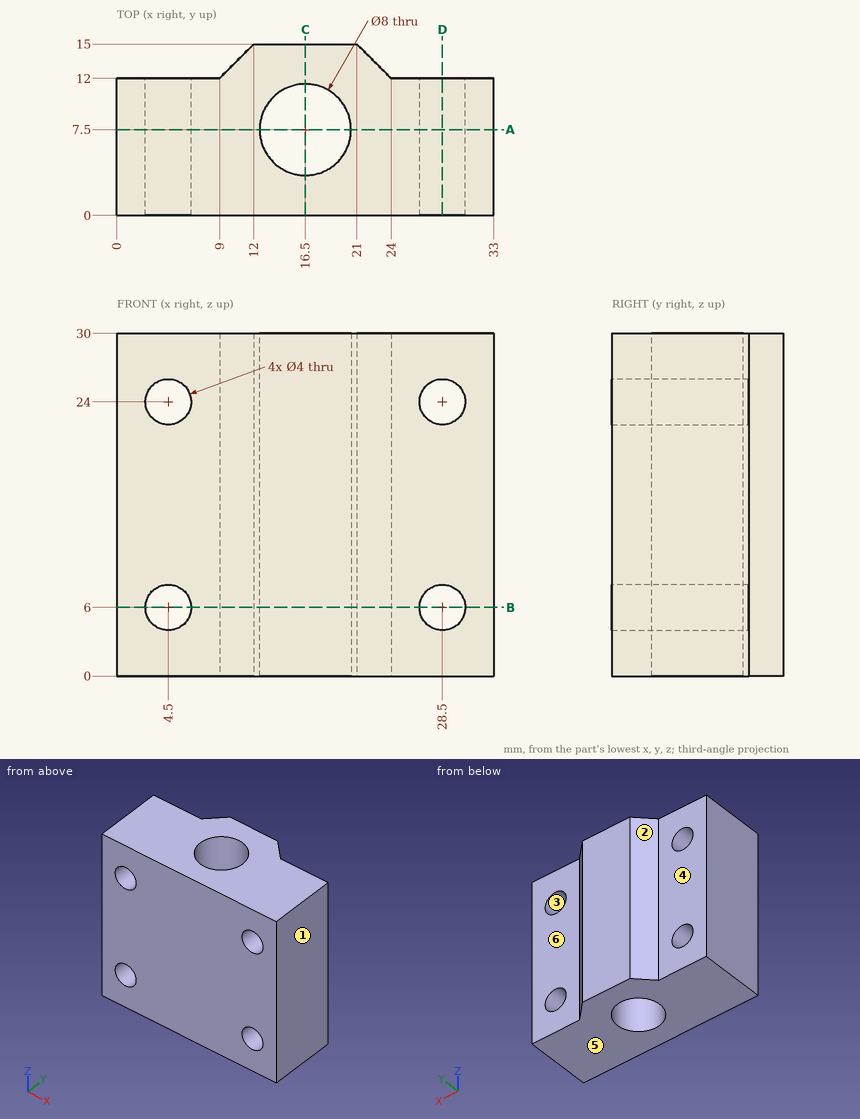
For this review, use the dimensioned drawing (mm, ordinates from the lowest corner) and the shaded views. A direction names the side the tool comes from. Round coordinates to 2 decimals unless told otherwise and drop trailing zeros. Loops run counter-clockwise (first coordinate to the right, second up) from the corner with the lowest first, then second, coordinate; pieces in that order, holes last. Notation, with made-up numbers: M -11,82.25 L 1,82.25 A13 cw 1,96.25 Z; hole C 22,-9 d7. An arc over 180 degrees is marked long. Answer as CSV lines item,"result".
1. We need section C-C (x = 16.5). Give the boundary of the cut face in (y, z).
Outcome:
outline,"M 0,0 L 3.5,0 L 3.5,30 L 0,30 Z; M 11.5,0 L 15,0 L 15,30 L 11.5,30 Z"
2. We need section B-B (z = 6). Give the boundary of the cut face in (x, y), plus the area to 3 significant figures.
Outcome:
outline,"M 0,0 L 2.5,0 L 2.5,12 L 0,12 Z; M 6.5,0 L 26.5,0 L 26.5,12 L 24,12 L 21,15 L 12,15 L 9,12 L 6.5,12 Z; M 30.5,0 L 33,0 L 33,12 L 30.5,12 Z; hole C 16.5,7.5 d8"
area,"286 mm2"
3. We need section A-A (y = 7.5). Give the boundary of the cut face in (x, z), plus the area to 3 significant figures.
Outcome:
outline,"M 0,0 L 12.5,0 L 12.5,30 L 0,30 Z; M 20.5,0 L 33,0 L 33,30 L 20.5,30 Z; hole C 4.5,6 d4; hole C 4.5,24 d4; hole C 28.5,6 d4; hole C 28.5,24 d4"
area,"700 mm2"
4. We need section D-D (x = 28.5). Give the boundary of the cut face in (y, z).
Outcome:
outline,"M 0,0 L 12,0 L 12,4 L 0,4 Z; M 0,8 L 12,8 L 12,22 L 0,22 Z; M 0,26 L 12,26 L 12,30 L 0,30 Z"
5. For the marked faces 4, 5 and 6, list the 3-axis set-ups (+Z, -Z, +X, -X, +Y, -Y) from which the entire face can be reached by the end or side of a thin tool; tool diameter is ignored.
Outcome:
face 4,"+Z, -Z, -X, +Y"
face 5,"-Z, +X, -X, +Y, -Y"
face 6,"+Z, -Z, +X, +Y"
6. Draft analysis for pull direction X (two halves, no side actions). For the marked faces 1, 2 and 3, state which applies: pulls with the +X half, pulls with the -X half, needs draft (parallel to the pull), parting line crosses it, or undercut.
Outcome:
face 1,"pulls with the +X half"
face 2,"pulls with the -X half"
face 3,"undercut"
7. To check wall thickness, follow L1, parallel to Z at x = 3, y = 6; L2, parallel to X at y = 8.5, z = 6; L3, parallel to Y at x = 23.5, z = 20. State the ranges of each line that lie inside material, in increasing order. Write a range as [from, to].
Outcome:
L1,"z = [0, 4.68], [7.32, 22.68], [25.32, 30]"
L2,"x = [0, 2.5], [6.5, 12.63], [20.37, 26.5], [30.5, 33]"
L3,"y = [0, 12.5]"
8. Insertion check: pin 1 Ø3.5 at (x, z) = (4.5, 6) entering from -Y; pin 2 Ø10 at (x, z) = (2.5, 17.5) entering from +Y; pin 3 Ø2 at (x, z) = (23, 26.5) entering from +Y. Each pin has a flat end and moves straight along its axis. Give the tip position at first contact, or say it passes through.
Outcome:
pin 1,"passes through"
pin 2,"stops at y = 12"
pin 3,"stops at y = 14"
